Autodesk Inventor part; units mm, degrees
ref_plane "YZ Plane" through (0, 0, 0) normal (1, 0, 0) x (0, 1, 0)
ref_plane "XZ Plane" through (0, 0, 0) normal (0, 1, 0) x (-1, 0, 0)
ref_plane "XY Plane" through (0, 0, 0) normal (0, 0, 1) x (1, 0, 0)
sketch "Sketch1" plane through (0, 0, 0) normal (0, 0, 1) x (1, 0, 0)
  circle A0 centre (-149.9998, -0.3235) radius 225 construction
  line L0 (0, 0) -> (0, 132.4058)
  line L1 (0, 132.4058) -> (17.5, 149.9058)
  line L2 (0, 132.4058) -> (24.7487, 132.4058) construction
  arc A1 (75, 0) -> (17.5, 149.9058) centre (-149.9998, -0.3235) ccw
  line L3 (75, 0) -> (25, 0)
  line L4 (25, 0) -> (17.5, 0)
  line L5 (0, 0) -> (7.5, 0)
  line L6 (7.5, 0) -> (7.5, -10)
  line L7 (7.5, -10) -> (17.5, -10)
  line L8 (17.5, -10) -> (17.5, 0)
  circle A2 centre (-149.9998, -0.3235) radius 200 construction
  line L9 (17.5, 149.9058) -> (17.5, 0)
  dimension "d0" = 75
  dimension "d1" = 450
  dimension "d3" = 45
  dimension "d37" = 50
  dimension "d38" = 7.5
  dimension "d39" = 7.5
  dimension "d40" = 10
  dimension "d41" = 25
  dimension "d79" = 149.9058
extrude "Extrusion1" add sketch "Sketch1" along normal blind 15
sketch "Sketch2" plane through (0, 0, 15) normal (0, 0, 1) x (1, 0, 0)
  circle A0 centre (58.4678, 25) radius 2.5
  circle A1 centre (56.1283, 39.8164) radius 2.5
  line L0 (0, 132.4058) -> (0, 0)
  line L1 (0, 0) -> (7.5, 0)
  line L2 (7.5, 0) -> (7.5, -10)
  line L3 (7.5, -10) -> (17.5, -10)
  line L4 (17.5, -10) -> (17.5, 0)
  line L5 (17.5, 0) -> (75, 0)
  arc A2 (75, 0) -> (17.5, 149.9058) centre (-149.9998, -0.3235) ccw
  line L6 (17.5, 149.9058) -> (0, 132.4058)
  arc A3 (59.4404, 15) -> (16.4825, 127.6751) centre (-149.9998, -0.3235) ccw construction
  line L7 (59.4404, 15) -> (17.5, 15) construction
  line L8 (17.5, 15) -> (15, 15) construction
  line L9 (15, 15) -> (15, 126.1926) construction
  line L10 (15, 126.1926) -> (16.4825, 127.6751) construction
  circle A4 centre (11.7593, 133.5945) radius 2.5
  circle A5 centre (-149.9998, -0.3235) radius 225 construction
  circle A6 centre (-149.9998, -0.3235) radius 210 construction
  dimension "d6" = 5
  dimension "d7" = 5
  dimension "d8" = 15
  dimension "d10" = 25
  dimension "d42" = 15
  dimension "d43" = 5
  dimension "d45" = 450
  dimension "d46" = 15
  dimension "d49" = 7.4745
extrude "Extrusion2" cut sketch "Sketch2" against normal through all contours A0 | A1 | A4
sketch "Sketch5" plane through (0, 0, 15) normal (0, 0, 1) x (1, 0, 0)
  line L0 (5, 137.4058) -> (12.0711, 130.3347)
  line L1 (5, 137.4058) -> (15, 137.4058) construction
  line L2 (12.0711, 130.3347) -> (15.6066, 133.8703)
  line L3 (15.6066, 133.8703) -> (8.5355, 140.9413)
  line L4 (8.5355, 140.9413) -> (5, 137.4058)
  line L5 (17.5, 149.9058) -> (0, 132.4058)
  point P0 (0, 0)
  dimension "d29" = 10
  dimension "d30" = 45
  dimension "d31" = 5
  dimension "d32" = 10
  dimension "d33" = 90
  dimension "d34" = 5
extrude "Extrusion3" cut sketch "Sketch5" against normal through all
thread "Thread1"
thread "Thread2"
thread "Thread3"
sketch "Sketch6" plane through (0, 0, 15) normal (0, 0, 1) x (1, 0, 0)
  line L0 (0, 107.4058) -> (20, 107.4058) construction
  line L1 (20, 107.4058) -> (20, 57.4058) construction
  line L2 (20, 57.4058) -> (0, 57.4058) construction
  line L3 (0, 57.4058) -> (0, 107.4058) construction
  line L4 (8.5355, 140.9413) -> (15.6066, 133.8703) construction
  line L5 (15.6066, 133.8703) -> (12.0711, 130.3347) construction
  line L6 (9.3094, 133.0964) -> (5, 137.4058) construction
  line L7 (5, 137.4058) -> (0, 132.4058) construction
  line L8 (0, 132.4058) -> (0, 0) construction
  line L9 (0, 0) -> (7.5, 0) construction
  line L10 (7.5, 0) -> (7.5, -10) construction
  line L11 (7.5, -10) -> (17.5, -10) construction
  line L12 (17.5, -10) -> (17.5, 0) construction
  line L13 (17.5, 0) -> (75, 0) construction
  arc A0 (75, 0) -> (17.5, 149.9058) centre (-149.9998, -0.3235) ccw construction
  line L14 (17.5, 149.9058) -> (8.5355, 140.9413) construction
  arc A1 (9.3094, 133.0964) -> (11.2612, 131.1446) centre (11.7593, 133.5945) ccw construction
  circle A2 centre (58.4678, 25) radius 2.5 construction
  circle A3 centre (56.1283, 39.8164) radius 2.5 construction
  circle A4 centre (10, 92.4058) radius 2.5
  circle A5 centre (10, 72.4058) radius 2.5
  line L15 (0, 132.4058) -> (0, 0)
  line L16 (12.0711, 130.3347) -> (11.2612, 131.1446)
  dimension "d50" = 20
  dimension "d51" = 50
  dimension "d52" = 25
  dimension "d53" = 5
  dimension "d54" = 5
  dimension "d55" = 20
  dimension "d56" = 15
  dimension "d57" = 10
extrude "Extrusion4" cut sketch "Sketch6" against normal through all
thread "Thread4"
thread "Thread5"
sketch "Sketch9" plane through (0, 0, 15) normal (0, 0, 1) x (1, 0, 0)
  line L0 (0, 132.4058) -> (0, 0)
  line L1 (0, 107.4058) -> (20, 107.4058)
  line L2 (20, 107.4058) -> (20, 57.4058)
  line L3 (20, 57.4058) -> (0, 57.4058)
  line L4 (0, 57.4058) -> (0, 107.4058)
  dimension "d74" = 20
  dimension "d75" = 50
  dimension "d76" = 25
extrude "Extrusion7" cut sketch "Sketch9" against normal blind 5
properties part number "CP001" material "ABS Plastic"
The listing builds one solid part. Answer for the finished solid, in the listing's coordinates (mm). A direction names the side the tool comes from. Coordinates: 2 decimals unless noted, no trailing zeros. Loops run counter-clockwise (first coordinate to the right, second up) from the corner with the lowest first, then second, coordinate; pieces in that order, holes last. Notation, with made-up numbers: (-17.5, -35) -> (31.5, -35) arc R33 cw to (31.5, -2) -> close; hole circle Ø3 at (-20.75, 69). An arc over 180 degrees is marked (long way). Return JSON: item names as keys, results as strings. Group by question number.
(1) A cutting plane is placed at B-B on y = 25. Write down the section's boundary in (x, z), and give its area (3 significant figures).
(2) A cutting plane is placed at C-C on z = 11.75. Write down the section's boundary in (x, y), and give its area (3 significant figures).
(3) Given pin 1 Ø3 at (x, y) = (58.47, 25) entering from +Z; pin 2 Ø10 at (x, y) = (14.5, 87) entering from +Z; pin 3 Ø6 at (y, z) = (87.5, 10.5) entering from +X; pin 4 Ø5 at (y, z) = (-3.5, 7.5) entering from +X, each flat-ended and moving along its own axis, determine where each tip first touches the part or whether it passes through.
(4) A cutting plane is placed at D-D on x = 41.5. Write down the section's boundary in (y, z).
(5) Which of the six approach directions +Z, -Z, +X, -X, +Y, -Y give full straight-line access (tool end or side, diameter ignored) to faces 4 (the flat face through (12.121, 137.356, 7.605)), 5 (the flat face through (17.5, -5, 7)), 6 (the flat face through (4, 0, 7)), 7 (the flat face through (10, 107.406, 13))?
(6) Find the intervals of material crossed by probe 1 along Y at (x, z) = (11.5, 2.5); probe 2 along Y at (x, z) = (10, 4); probe 3 along Z at (x, y) = (15.5, 71), in increasing order. Write a range as from..to.
(7) Determine the mould class of faces 1 (the flat face through (37, 53, 15)), 2 (the flat face through (13.814, 132.078, 7.605)), 3 (the flat face through (2.465, 134.871, 7.395)) for opening direction X: released by +X, released by -X, zero draft, split by the parting line, or undercut.
(8) A cutting plane is placed at A-A on z = 4.75. Write down the section's boundary in (x, y), and give its area (3 significant figures).
The answers:
{
 "1": {"outline": "(0, 0) -> (55.97, 0) -> (55.97, 15) -> (0, 15) -> close; (60.97, 0) -> (73.57, 0) -> (73.57, 15) -> (60.97, 15) -> close", "area": "1,030 mm^2"},
 "2": {"outline": "(0, 0) -> (7.5, 0) -> (7.5, -10) -> (17.5, -10) -> (17.5, 0) -> (75, 0) arc R225 ccw to (17.5, 149.91) -> (8.54, 140.94) -> (15.61, 133.87) -> (12.07, 130.33) -> (11.26, 131.14) arc R2.5 cw to (9.31, 133.1) -> (5, 137.41) -> (0, 132.41) -> (0, 107.41) -> (20, 107.41) -> (20, 57.41) -> (0, 57.41) -> close; hole circle Ø5 at (56.13, 39.82); hole circle Ø5 at (58.47, 25)", "area": "7,390 mm^2"},
 "3": {"pin 1": "passes through", "pin 2": "stops at z = 10", "pin 3": "stops at x = 58.4", "pin 4": "stops at x = 17.5"},
 "4": {"outline": "(0, 0) -> (117.8, 0) -> (117.8, 15) -> (0, 15) -> close"},
 "5": {"face 4": "+Z, -Z", "face 5": "+Z, -Z, +X, -Y", "face 6": "+Z, -Z, -X, -Y", "face 7": "+Z, -X"},
 "6": {"probe 1": "y = -10..70.41, 74.41..90.41, 94.41..130.91, 137.98..143.91", "probe 2": "y = -10..69.91, 74.91..89.91, 94.91..131.82, 139.48..142.41", "probe 3": "z = 0..10"},
 "7": {"face 1": "zero draft", "face 2": "undercut", "face 3": "released by -X"},
 "8": {"outline": "(0, 0) -> (7.5, 0) -> (7.5, -10) -> (17.5, -10) -> (17.5, 0) -> (75, 0) arc R225 ccw to (17.5, 149.91) -> (8.54, 140.94) -> (15.61, 133.87) -> (12.07, 130.33) -> (11.26, 131.14) arc R2.5 cw to (9.31, 133.1) -> (5, 137.41) -> (0, 132.41) -> close; hole circle Ø5 at (10, 72.41); hole circle Ø5 at (10, 92.41); hole circle Ø5 at (56.13, 39.82); hole circle Ø5 at (58.47, 25)", "area": "8,350 mm^2"}
}
